Can you work these out from the model? Positions are in its coordinate system, mm. Face numbers are marked on the shaded views. A direction names the side the tool comes from. Round coordinates to 2 decimals unless told otherwise and drop trailing zeros. Write each loop counter-clockwise with the first axis right and the second up, starting at its lowest first coordinate (ties: lowest second). Pieces come first, ordered by that corner, then holes. Notation, with made-up numbers: M 0.5,57 L 50.5,57 A20 ccw 50.5,91 Z; hole C -30,13 d9. An arc over 180 degrees is marked long. Answer in a Markdown table with one row per item. Add a question column.
(1) Suppose I cut it at B-B, the plane y = 34.5. Write out the boundary of the cut face in (x, z), then the cut area to 3 significant figures.
(2) I'm going to push flat-ended pins straight in: pin 1 (1.9 mm diameter, centred on y = 2.44, z = 11.25, fed in from +X); pin 2 (2.5 mm diameter, centred on x = -1, y = 24, fed in from +Z). Where does each tip first touch, or does it pass through?
(3) For the marked faces 1 and 2, which set-ups out of +Z, -Z, +X, -X, +Y, -Y let a thin tool reach every point of the face, with its end or its side?
(4) Suppose I cut it at C-C, the plane x = 0.6. Count the separate pieces of the cut face and the enclosed holes in it, then the cut area to 3 significant figures.
(5) If we mould it in two halves opening along Z, with no side actions, what happens to the marked faces 3, 4 and 5? For each: released by +Z, released by -Z, zero draft, split by the parting line, or undercut.
(6) If I drill on probe 1 along Z at (x, y) = (-0.6, 16); probe 2 along Z at (x, y) = (0.5, 13.5); probe 3 along Z at (x, y) = (1.55, 44), over which ranges is the centre line in solid material (lowest first)?
(7) Suppose I cut it at D-D, the plane z = -11.25. Write out the boundary of the cut face in (x, y), then the cut area to 3 significant figures.
(8) Suppose I cut it at A-A, the plane z = 0. Write out the boundary of the cut face in (x, y), then the cut area to 3 significant figures.
from build123d import *

# Parameters (mm, degrees)
BOSS_EXTRUDE1_DEPTH       = 2.3815
M3_CLEARANCE_HOLE1_D      = 3.2
F_1_0MM_START             = -2.3815
F_1_0MM_DOWEL_SLOT1_DEPTH = 4.763


# Read off the part's stored shape, not the designer's step: Ø1.0mm Dowel Slot1
with BuildPart() as part:
    # Sketch1 → Boss-Extrude1 (new, symmetric)
    with BuildSketch(Plane(origin=(0, 0, 0), x_dir=(0, 0, -1), z_dir=(1, 0, 0))):
        with BuildLine():
            Line((-22.5, 0), (22.5, 0))
            Line((22.5, 0), (22.5, 4.873))
            Line((22.5, 4.873), (4.655163533, 62.882072013))
            ThreePointArc((4.655163533, 62.882072013), (3.570153218, 64.413111688), (1.787769426, 65))
            Line((1.787769426, 65), (-1.787769426, 65))
            ThreePointArc((-1.787769426, 65), (-3.570795025, 64.412637502), (-4.655632377, 62.880546477))
            Line((-4.655632377, 62.880546477), (-22.5, 4.763))
            Line((-22.5, 4.763), (-22.5, 0))
        make_face()
        with BuildLine():
            Line((6.507919955, 11.613028191), (6.507919955, 29.434537867))
            ThreePointArc((6.507919955, 29.434537867), (7.858931987, 31.004324378), (9.612461298, 29.90223629))
            Line((9.612461298, 29.90223629), (15.094257994, 12.121307765))
            ThreePointArc((15.094257994, 12.121307765), (14.833637596, 10.588440441), (13.445586349, 9.887784348))
            Line((13.445586349, 9.887784348), (8.233163799, 9.887784348))
            ThreePointArc((8.233163799, 9.887784348), (7.013232178, 10.39309657), (6.507919955, 11.613028191))
        make_face(mode=Mode.SUBTRACT)
        with BuildLine():
            Line((-9.612461298, 29.90223629), (-15.094257994, 12.121307765))
            ThreePointArc((-15.094257994, 12.121307765), (-14.833637596, 10.588440441), (-13.445586349, 9.887784348))
            Line((-13.445586349, 9.887784348), (-8.233163799, 9.887784348))
            ThreePointArc((-8.233163799, 9.887784348), (-7.013232178, 10.39309657), (-6.507919955, 11.613028191))
            Line((-6.507919955, 11.613028191), (-6.507919955, 29.434537867))
            ThreePointArc((-6.507919955, 29.434537867), (-7.858931987, 31.004324378), (-9.612461298, 29.90223629))
        make_face(mode=Mode.SUBTRACT)
    extrude(amount=BOSS_EXTRUDE1_DEPTH, both=True)

    # M3 Clearance Hole1 (through all)
    with Locations(Plane(origin=(2.3815, 0, 0), x_dir=(0, 0, -1), z_dir=(1, 0, 0))):
        with Locations((11.25, 2.4365), (-11.250134442, 2.436499343)):
            Hole(M3_CLEARANCE_HOLE1_D / 2)

    # Ø1.0mm Dowel Slot1 outline → Ø1.0mm Dowel Slot1 (cut)
    with BuildSketch(Plane.YZ.offset(F_1_0MM_START)):
        with BuildLine():
            Line((12.367584087, -2.520038343), (42.366612584, -2.761469965))
            ThreePointArc((42.366612584, -2.761469965), (44.886650928, -0.281670226), (42.406851188, 2.238368118))
            Line((42.406851188, 2.238368118), (12.407822691, 2.47979974))
            ThreePointArc((12.407822691, 2.47979974), (9.887784348, 0), (12.367584087, -2.520038343))
        make_face()
    extrude(amount=F_1_0MM_DOWEL_SLOT1_DEPTH, mode=Mode.SUBTRACT)


solid = part.part
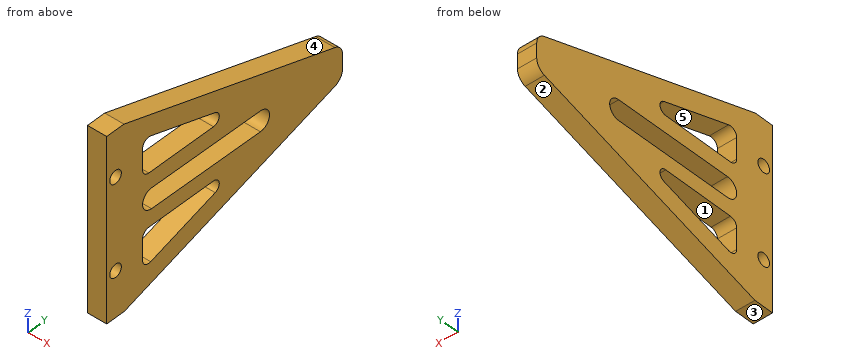
Calculated:
| question | item | result |
|---|---|---|
| 1 | outline | M -2.38,-13.39 L 2.38,-13.39 L 2.38,-2.7 L -2.38,-2.7 Z; M -2.38,2.3 L 2.38,2.3 L 2.38,13.37 L -2.38,13.37 Z |
| 1 | area | 104 mm² |
| 2 | pin 1 | through |
| 2 | pin 2 | z = 16.98 |
| 3 | face 1 | +X, -X |
| 3 | face 2 | -Z, +X, -X, +Y |
| 4 | separate pieces | 1 |
| 4 | enclosed holes | 5 |
| 4 | area | 1,380 mm² |
| 5 | face 3 | released by -Z |
| 5 | face 4 | released by +Z |
| 5 | face 5 | undercut |
| 6 | probe 1 | -19.08 to -13.9, -6.51 to -2.55, 2.45 to 6.51, 13.9 to 19.05 |
| 6 | probe 2 | -19.85 to -14.67, -6.51 to -2.53, 2.47 to 6.51, 14.67 to 19.82 |
| 6 | probe 3 | -10.46 to -2.17, 1.65 to 10.45 |
| 7 | outline | M -2.38,0 L 2.38,0 L 2.38,0.84 L -2.38,0.84 Z; M -2.38,4.04 L 2.38,4.04 L 2.38,9.89 L -2.38,9.89 Z; M -2.38,24.59 L 2.38,24.59 L 2.38,41.44 L -2.38,41.44 Z |
| 7 | area | 112 mm² |
| 8 | outline | M -2.38,0 L 2.38,0 L 2.38,9.89 L -2.38,9.89 Z; M -2.38,44.87 L 2.38,44.87 L 2.38,65 L -2.38,65 Z |
| 8 | area | 143 mm² |
